Design review of the part shown in the three views and the two pictorial views. Dimensions are in mm from the part's minimum x, y and z. Coordinates: 2 decimals unless noted, no trailing zeros. Write each loop counter-clockwise with the first axis right and the second up, starting at its lowest first coordinate (ties: lowest second). Pieces come first, ordered by that corner, then holes. Notation, with made-up numbers: (52, 50.25) - (95, 50.25) arc R20 cw to (95, 80.25) - close; hole circle Ø9 at (62, -32). An arc over 180 degrees is marked (long way). Write each question's results on one line, items separated by ' | '.
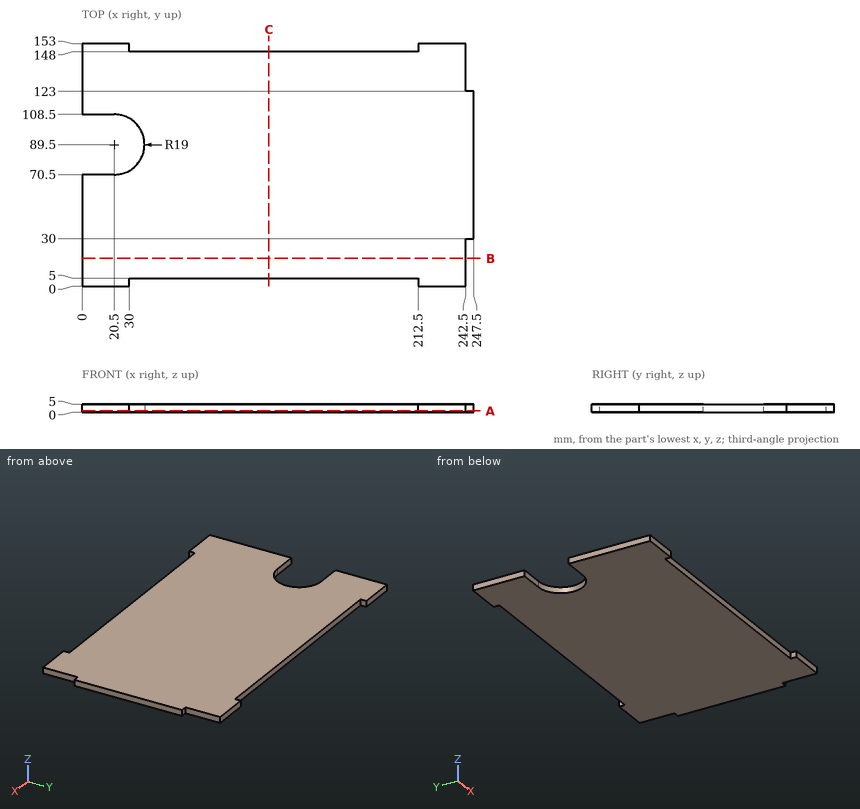
Q1. For pin 1 (1.5 mm diameter, centred on x = 244.5, z = 2, fed in from +Y); pin 2 (1.5 mm diameter, centred on y = 13, z = 2, fed in from +X); pin 3 (1.5 mm diameter, centred on x = 79, z = 3.5, fed in from -Y), all flat-tipped, find the tip position at first contact; note any pin that passes through.
Results found:
pin 1: y = 123 | pin 2: x = 242.5 | pin 3: y = 5
Q2. Wall thickness on line 1 along Y through (x, z) = (18, 1.3); line 2 along Y through (x, z) = (56, 1.6); line 3 along Y through (x, z) = (28, 3.65): over which ranges is each line inside the solid? List them lowest first. Write a range as from..to.
Results found:
line 1: 0..70.5, 108.5..153 | line 2: 5..148 | line 3: 0..72.04, 106.96..153
Q3. Take a section at B-B on y = 17.5. State the section outline as (x, z) points, plus the area to 3 significant figures.
Results found:
outline: (0, 0) - (242.5, 0) - (242.5, 5) - (0, 5) - close | area: 1,210 mm2
Q4. Take a section at C-C on x = 118. State the section outline as (y, z) points, plus the area to 3 significant figures.
Results found:
outline: (5, 0) - (148, 0) - (148, 5) - (5, 5) - close | area: 715 mm2
Q5. Take a section at A-A on z = 0.85. State the section outline as (x, y) points, plus the area to 3 significant figures.
Results found:
outline: (0, 0) - (30, 0) - (30, 5) - (212.5, 5) - (212.5, 0) - (242.5, 0) - (242.5, 30) - (247.5, 30) - (247.5, 123) - (242.5, 123) - (242.5, 153) - (212.5, 153) - (212.5, 148) - (30, 148) - (30, 153) - (0, 153) - (0, 108.5) - (20.5, 108.5) arc R19 cw to (20.5, 70.5) - (0, 70.5) - close | area: 34,400 mm2
